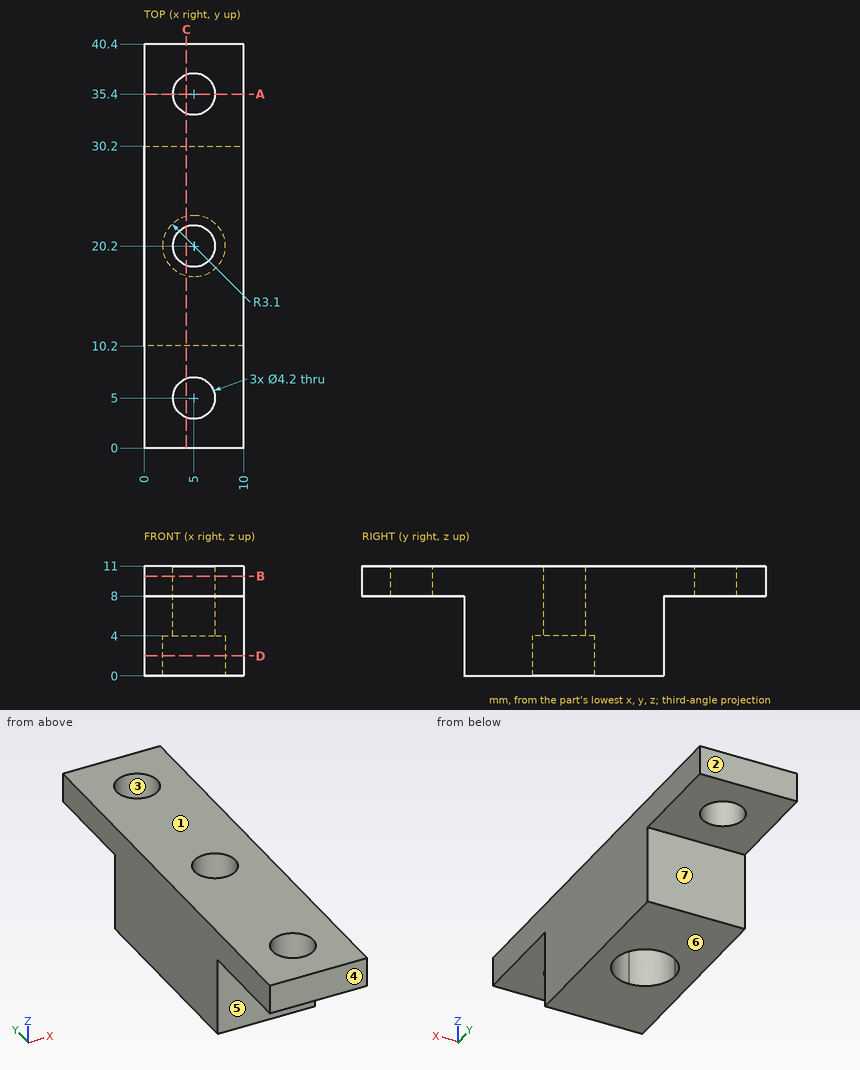
Answer from the drawing. Dimensions are ordinates in mm from the lowest x, y and z of the part. A direction names the side the tool comes from. Round coordinates to 2 decimals unless told otherwise and drop trailing zeros. Write each loop counter-clockwise with the first axis right and the second up, starting at its lowest first coordinate (ties: lowest second). Pieces come first, ordered by that corner, then holes. Notation, with made-up numbers: (39.25, 15.5) - (98.25, 15.5) arc R19 cw to (98.25, 30.5) - close; hole circle Ø1 at (40.5, -38). An arc over 180 degrees is marked (long way). One line per item, written item: value.
Q1. Straight lines are drawn through the part: line 1 (Y direction, x = 5, z = 9.95); line 2 (X direction, y = 5, z = 9); line 3 (Y direction, x = 1.25, z = 2). For each, find the intervals that lie inside material, in ascending order. Write a range as from..to.
The answers:
line 1: y = 0..2.9, 7.1..18.1, 22.3..33.3, 37.5..40.4
line 2: x = 0..2.9, 7.1..10
line 3: y = 10.2..30.2
Q2. Find section C-C (x = 4.25). Determine the outline of the cut face in (y, z), and give its area (3 significant figures).
The answers:
outline: (0, 8) - (3.04, 8) - (3.04, 11) - (0, 11) - close; (6.96, 8) - (10.2, 8) - (10.2, 0) - (17.19, 0) - (17.19, 4) - (18.24, 4) - (18.24, 11) - (6.96, 11) - close; (22.16, 4) - (23.21, 4) - (23.21, 0) - (30.2, 0) - (30.2, 8) - (33.44, 8) - (33.44, 11) - (22.16, 11) - close; (37.36, 8) - (40.4, 8) - (40.4, 11) - (37.36, 11) - close
area: 206 mm2
Q3. For a pull along Y with two mould halves and no side action, classify the marked faces 1, 2, 3 and 4 as pulls with the +Y half, pulls with the -Y half, needs draft (parallel to the pull), parting line crosses it, or undercut.
The answers:
face 1: needs draft
face 2: pulls with the +Y half
face 3: undercut
face 4: pulls with the -Y half
Q4. Each of these flat-tipped pins is pushed along its axis until it touches: P1, Ø4, axis at x = 5.5, z = 5.5, coming from the +Y side; P2, Ø2.5, axis at x = 5, y = 5, coming from the -Z side (3 decimals); P3, Ø5, axis at x = 5, y = 6, coming from the -Z side; P4, Ø1, axis at x = 2, z = 4, coming from the -Y side. Where does it stop, or does it pass through?
The answers:
P1: stops at y = 30.2
P2: passes through
P3: stops at z = 8
P4: stops at y = 10.2
Q5. Which of the six approach directions +Z, -Z, +X, -X, +Y, -Y give full straight-line access (tool end or side, diameter ignored) to the marked faces 5, 6 and 7?
The answers:
face 5: -Z, +X, -X, -Y
face 6: -Z, +X, -X, +Y, -Y
face 7: -Z, +X, -X, +Y
Q6. Find section B-B (z = 10). Determine the outline of the cut face in (x, y).
The answers:
outline: (0, 0) - (10, 0) - (10, 40.4) - (0, 40.4) - close; hole circle Ø4.2 at (5, 5); hole circle Ø4.2 at (5, 20.2); hole circle Ø4.2 at (5, 35.4)
Q7. Find section A-A (y = 35.4). Determine the outline of the cut face in (x, z), and give its area (3 significant figures).
The answers:
outline: (0, 8) - (2.9, 8) - (2.9, 11) - (0, 11) - close; (7.1, 8) - (10, 8) - (10, 11) - (7.1, 11) - close
area: 17.4 mm2
Q8. Find section D-D (z = 2). Determine the outline of the cut face in (x, y).
The answers:
outline: (0, 10.2) - (10, 10.2) - (10, 30.2) - (0, 30.2) - close; hole circle Ø6.2 at (5, 20.2)
